```python
from build123d import *

# Parameters (mm, degrees)
SPEAKERMOUNTING_W               = 227.80625
SPEAKERMOUNTING_H               = 182.5625
SPEAKERMOUNTING_THICKNESS_DEPTH = 11.43
SPEAKERCUTOUT_R                 = 1.5875
SPEAKERCUTOUT_RX                = 93.6625
SPEAKERCUTOUT_RY                = 65.087499997
CUT_EXTRUDE1_DEPTH              = 11.43
CUT_EXTRUDE2_DEPTH              = 227.80625
SKETCH2_R                       = 1.5875
CUT_EXTRUDE3_DEPTH              = 11.43


with BuildPart() as part:
    # SpeakerMounting → SpeakerMounting_Thickness (new body)
    with BuildSketch(Plane.XY):
        with Locations((-5626.496875, 1089.81875)):
            Rectangle(SPEAKERMOUNTING_W, SPEAKERMOUNTING_H)
    extrude(amount=-SPEAKERMOUNTING_THICKNESS_DEPTH)

    # SpeakerCutout → Cut-Extrude1 (cut)
    with BuildSketch(Plane.XY):
        with Locations((-5571.33125, 1153.31875)):
            Circle(SPEAKERCUTOUT_R)
        with Locations((-5518.94375, 1155.7)):
            Circle(SPEAKERCUTOUT_R)
        with Locations((-5518.94375, 1023.9375)):
            Circle(SPEAKERCUTOUT_R)
        with Locations((-5550.69375, 1004.8875)):
            Circle(SPEAKERCUTOUT_R)
        with Locations((-5571.33125, 1026.31875)):
            Circle(SPEAKERCUTOUT_R)
        with Locations((-5679.28125, 1026.31875)):
            Circle(SPEAKERCUTOUT_R)
        with Locations((-5702.3, 1004.8875)):
            Circle(SPEAKERCUTOUT_R)
        with Locations((-5679.28125, 1153.31875)):
            Circle(SPEAKERCUTOUT_R)
        with Locations(Location((-5625.30625, 1089.81875), (0, 0, 180))):
            Ellipse(SPEAKERCUTOUT_RX, SPEAKERCUTOUT_RY)
    extrude(amount=-CUT_EXTRUDE1_DEPTH, mode=Mode.SUBTRACT)

    # SpeakerSlotForScreen → Cut-Extrude2 (cut)
    with BuildSketch(Plane(origin=(-5512.59375, 0, 0), x_dir=(0, 0, -1), z_dir=(1, 0, 0))):
        Polygon((5.715, 1181.1), (3.175, 1181.1), (3.175, 1174.75), (9.525, 1174.75), (9.525, 1181.1), align=None)
    extrude(amount=-CUT_EXTRUDE2_DEPTH, mode=Mode.SUBTRACT)

    # Sketch2 → Cut-Extrude3 (cut)
    with BuildSketch(Plane(origin=(0, 0, -11.43), x_dir=(-1, 0, 0), z_dir=(0, 0, -1))):
        with Locations((5729.43355, 1004.8875)):
            Circle(SKETCH2_R)
    extrude(amount=-CUT_EXTRUDE3_DEPTH, mode=Mode.SUBTRACT)


solid = part.part
```
Geometry check sheet. Reference: the model listing, model coordinates, mm. A direction names the side the tool comes from. Round coordinates to 2 decimals unless told otherwise and drop trailing zeros. Use a Markdown table: item, result.
Q1. Access from +Z, -Z, +X, -X, +Y, -Y to the whole of each face (thin tool, end or side, straight path). Record for faces 1 (the flat face through (-5625, 1174.75, -6)), 2 (the flat face through (-5679, 1030, 0)).
Solutions:
| item | result |
|---|---|
| face 1 | +X, -X, +Y |
| face 2 | +Z, +X, -X, +Y, -Y |
Q2. Draft check along Z on faces 3 (the flat face through (-5679, 1030, -11.43)), 4 (the flat face through (-5512.594, 1089, -6)), 5 (the flat face through (-5625, 1178, -9.525)). Enter one of: released by +Z, released by -Z, zero draft, split by the parting line, or undercut.
Solutions:
| item | result |
|---|---|
| face 3 | released by -Z |
| face 4 | zero draft |
| face 5 | undercut |
Q3. Material ranges on line 1 (X direction, y = 1137.5, z = -11); line 2 (X direction, y = 1125.5, z = -6); line 3 (Y direction, x = -5589.5, z = -10.5), recorded low to high.
Solutions:
| item | result |
|---|---|
| line 1 | x = -5740.4 to -5689.06, -5561.55 to -5512.59 |
| line 2 | x = -5740.4 to -5703.64, -5546.97 to -5512.59 |
| line 3 | y = 998.54 to 1029.68, 1149.96 to 1181.1 |
Q4. Go/stop test with flat-tipped pins: P1, Ø2.5, axis at x = -5550.69, y = 1004.89, coming from the -Z side; P2, Ø1.9, axis at x = -5667.5, z = -6.5, coming from the +Y side. Record where each tip stops, or that it passes through.
Solutions:
| item | result |
|---|---|
| P1 | passes through |
| P2 | stops at y = 1174.75 |
